```python
from build123d import *

# Parameters (mm, degrees)
F0_W           = 50
F0_H           = 50
F1_DEPTH       = 5
F3_D           = 5
F3_CSINK_D     = 8
F3_CSINK_ANGLE = 90
F4_R           = 23.40982
F5_DEPTH       = 25
F7_D           = 5
F7_CSINK_D     = 8
F7_CSINK_ANGLE = 90
F8_R           = 3.742028
F9_DEPTH       = 25


with BuildPart() as f1:
    # F0 (on Top) → F1 (new body)
    with BuildSketch(Plane.XY):
        Rectangle(F0_W, F0_H)
    extrude(amount=F1_DEPTH)

    # F3 (through all)
    with Locations(Plane.XY.offset(5)):
        with Locations((0, 17.408038), (15.075803, 8.704019), (15.075803, -8.704019), (0, -17.408038), (-15.075803, -8.704019), (-15.075803, 8.704019)):
            CounterSinkHole(F3_D / 2, F3_CSINK_D / 2, counter_sink_angle=F3_CSINK_ANGLE)

    # F4 (on face) → F5 (intersect)
    with BuildSketch(Plane.XY.offset(5)):
        Circle(F4_R)
    extrude(amount=-F5_DEPTH, mode=Mode.INTERSECT)

    # F7 (through all)
    with Locations(Plane.XY.offset(5)):
        with Locations((-5.298098, 9.176576), (5.298098, 9.176576), (10.596197, 0), (5.298098, -9.176576), (-5.298098, -9.176576), (-10.596197, 0)):
            CounterSinkHole(F7_D / 2, F7_CSINK_D / 2, counter_sink_angle=F7_CSINK_ANGLE)

    # F8 (on face) → F9 (join)
    with BuildSketch(Plane.XY.offset(5)):
        Circle(F8_R)
    extrude(amount=F9_DEPTH)


solid = f1.part
```
CAD build for the part. Positions are in the model's coordinates, mm. A direction names the side the tool comes from. Coordinates: 2 decimals unless noted, no trailing zeros. Order: outer loops, then holes, each group sorted by start corner. A loop starts at its lowest first (then second) coordinate and runs counter-clockwise, first axis right, second up. Notation, with made-up numbers: (52, 39.5) -> (97, 39.5) arc R26 ccw to (97, 55.5) -> close; hole circle Ø6 at (89.25, 83.5). An arc over 180 degrees is marked (long way). Use one line per item in the form item = value. Start each with the question number.
1) Band-saw the part on D-D on z = 16. Give the cut face in (x, y), then the cut area to 3 significant figures.
2) Band-saw the part on B-B on y = 0. Give the cut face in (x, z).
3) Band-saw the part on A-A on x = 0. Give the cut face in (y, z), then the cut area to 3 significant figures.
4) Drop flat-ended pins along their axis: pin 1 (12 mm diameter, centred on x = 13, y = -14.5, fed in from +Z); pin 2 (6 mm diameter, centred on x = -15.08, y = -8.7, fed in from +Z); pin 3 (3 mm diameter, centred on x = 5.3, y = -9.18, fed in from +Z); pin 4 (3 mm diameter, centred on y = 6, z = 6, fed in from -X). Give the stop position or say it passes through.
5) Band-saw the part on C-C on y = -10. State how many separate pieces and enclosed holes the cut face has, then the cut area to 3 significant figures.
6) Drill centre lines: L1, parallel to Y at x = 0, z = 2.05; L2, parallel to Y at x = -4.5, z = 2.75; L3, parallel to X at y = -11, z = 3.75. Where is each one in solid material? Low to high. Write a range as [from, to].
7) Tool access for faces 4 (the cylindrical face through (-2.97, -2.277, 17.325)), 5 (the cylindrical face through (12.69, 9.45, 1.73)): list every direction of +Z, -Z, +X, -X, +Y, -Y with a clear straight run to the whole face (end or side of a thin tool).
8) Pull direction Y, two halves, no side cores. Call faces 1 (the cylindrical face through (-23.387, 1.029, 2.535)), 2 (the flat face through (0, 0, 30)), 3 (the cylindrical face through (15.618, -11.145, 1.725)): +Y half, -Y half, draft (parallel to the pull), parting line (faces both ways), or undercut.
Entries:
q1.outline = circle Ø7.48 at (0, 0)
q1.area = 44.0 mm2
q2.outline = (-23.41, 0) -> (-13.1, 0) -> (-13.1, 3.5) -> (-14.6, 5) -> (-23.41, 5) -> close; (-8.1, 0) -> (8.1, 0) -> (8.1, 3.5) -> (6.6, 5) -> (3.74, 5) -> (3.74, 30) -> (-3.74, 30) -> (-3.74, 5) -> (-6.6, 5) -> (-8.1, 3.5) -> close; (13.1, 0) -> (23.41, 0) -> (23.41, 5) -> (14.6, 5) -> (13.1, 3.5) -> close
q3.outline = (-23.41, 0) -> (-19.91, 0) -> (-19.91, 3.5) -> (-21.41, 5) -> (-23.41, 5) -> close; (-14.91, 0) -> (14.91, 0) -> (14.91, 3.5) -> (13.41, 5) -> (3.74, 5) -> (3.74, 30) -> (-3.74, 30) -> (-3.74, 5) -> (-13.41, 5) -> (-14.91, 3.5) -> close; (19.91, 0) -> (23.41, 0) -> (23.41, 5) -> (21.41, 5) -> (19.91, 3.5) -> close
q3.area = 367 mm2
q4.pin_1 = 5
q4.pin_2 = 4.01
q4.pin_3 = through
q4.pin_4 = -22.9
q5.separate_pieces = 5
q5.enclosed_holes = 0
q5.area = 112 mm2
q6.L1 = [-23.41, -19.91], [-14.91, 14.91], [19.91, 23.41]
q6.L2 = [-22.97, -11.55], [-6.81, 6.81], [11.55, 22.97]
q6.L3 = [-20.66, -16.59], [-13.56, -7.36], [-3.24, 3.24], [7.36, 13.56], [16.59, 20.66]
q7.face_4 = +Z
q7.face_5 = +Z, -Z
q8.face_1 = parting line
q8.face_2 = draft
q8.face_3 = undercut
